Can you work these out from the model? Positions are in its coordinate system, mm. A direction names the side the tool comes from. Give positions to 0.01 mm unless a question says otherwise; leave off trailing zeros. Loops run counter-clockwise (first coordinate to the right, second up) from the corner with the lowest first, then second, coordinate; pieces in that order, holes last. Notation, with made-up numbers: (-20, -18.5) -> (37, -18.5) arc R7 ccw to (37, -5.5) -> close; hole circle Ø10 at (-35.5, 59.5). An arc over 180 degrees is marked (long way). Return JSON: item names as keys, results as strings. Group by question number.
Q1. I need wall thicknesses on line 1 along Z through (x, y) = (85, 1.75); line 2 along X through (y, z) = (2.95, -19); line 3 along X through (y, z) = (2.45, -25). Which ranges of each line are inside material? Lowest first, please. Write a range as [from, to].
Q2. Suppose I cut it at A-A, the plane x = 80.7. Please give me the cut outline in (y, z), and give its area (3 significant figures).
Q3. Which directions (+Z, -Z, +X, -X, +Y, -Y) give clear straight access to the entire face, cutting with the end or side of a thin tool? Please do faces 1 (the flat face through (59.7, 2, 0)), 2 (the flat face through (-1, 2, -60)).
Q4. Suppose I cut it at C-C, the plane y = 2.3. Count the separate pieces of the cut face and the enclosed holes in it, and give its area (3 significant figures).
Q5. Thinking about a two-plate mould opening in X: for faces 3 (the flat face through (-90, 2, 1)), 4 (the flat face through (39, 2, 15)), 5 (the flat face through (-1, 0, -1)), which applies, pulls with the +X half, pulls with the -X half, needs draft (parallel to the pull), parting line crosses it, or undercut?
Q6. Suppose I cut it at B-B, the plane z = -1. Please give me the cut outline in (x, y).
```python
from build123d import *

# Parameters (mm, degrees)
SKETCH_1_W          = 180
SKETCH_1_H          = 120
EXTRUDE_1_DEPTH     = 4
SKETCH_2_R          = 1.6
SKETCH_2_R_2        = 3
CUT_EXTRUDE_1_DEPTH = 4
SKETCH_3_W          = 40
SKETCH_3_H          = 30
CUT_EXTRUDE_2_DEPTH = 4
SKETCH_4_R          = 1.6
CUT_EXTRUDE_3_DEPTH = 4
SKETCH_5_R          = 1.6
CUT_EXTRUDE_4_DEPTH = 4


with BuildPart() as part:
    # 草图1 → 凸台-拉伸1 (new body)
    with BuildSketch(Plane(origin=(0, 0, 0), x_dir=(1, 0, 0), z_dir=(0, 1, 0))):
        Rectangle(SKETCH_1_W, SKETCH_1_H)
    extrude(amount=EXTRUDE_1_DEPTH)

    # 草图2 → 切除-拉伸1 (cut)
    with BuildSketch(Plane(origin=(0, 4, 0), x_dir=(1, 0, 0), z_dir=(0, 1, 0))):
        with Locations(Location((66, 25, 0), (0, 0, 270))):
            Circle(SKETCH_2_R)
        with Locations(Location((66, -25, 0), (0, 0, 270))):
            Circle(SKETCH_2_R)
        with Locations(Location((85, -25, 0), (0, 0, 270))):
            Circle(SKETCH_2_R)
        with Locations(Location((85, 25, 0), (0, 0, 270))):
            Circle(SKETCH_2_R)
        with Locations(Location((80.7, 7, 0), (0, 0, 270))):
            Circle(SKETCH_2_R_2)
    extrude(amount=-CUT_EXTRUDE_1_DEPTH, mode=Mode.SUBTRACT)

    # 草图3 → 切除-拉伸2 (cut)
    with BuildSketch(Plane(origin=(0, 4, 0), x_dir=(1, 0, 0), z_dir=(0, 1, 0))):
        with Locations((39.7, 0)):
            Rectangle(SKETCH_3_W, SKETCH_3_H)
    extrude(amount=-CUT_EXTRUDE_2_DEPTH, mode=Mode.SUBTRACT)

    # 草图4 → 切除-拉伸3 (cut)
    with BuildSketch(Plane(origin=(0, 4, 0), x_dir=(1, 0, 0), z_dir=(0, 1, 0))):
        with Locations(Location((-27.3, 56, 0), (0, 0, 270))):
            Circle(SKETCH_4_R)
        with Locations(Location((9.7, 56, 0), (0, 0, 270))):
            Circle(SKETCH_4_R)
        with Locations(Location((9.7, 19, 0), (0, 0, 270))):
            Circle(SKETCH_4_R)
        with Locations(Location((-27.3, 19, 0), (0, 0, 270))):
            Circle(SKETCH_4_R)
    extrude(amount=-CUT_EXTRUDE_3_DEPTH, mode=Mode.SUBTRACT)

    # 草图5 → 切除-拉伸4 (cut)
    with BuildSketch(Plane(origin=(0, 4, 0), x_dir=(1, 0, 0), z_dir=(0, 1, 0))):
        with Locations(Location((-39.8, -7.8, 0), (0, 0, 270))):
            Circle(SKETCH_5_R)
        with Locations(Location((9.7, -23, 0), (0, 0, 270))):
            Circle(SKETCH_5_R)
        with Locations(Location((9.7, -50.9, 0), (0, 0, 270))):
            Circle(SKETCH_5_R)
        with Locations(Location((-41.1, -56, 0), (0, 0, 270))):
            Circle(SKETCH_5_R)
    extrude(amount=-CUT_EXTRUDE_4_DEPTH, mode=Mode.SUBTRACT)


solid = part.part
```
Ans:
{
 "1": {"line 1": "z = [-60, -26.6], [-23.4, 23.4], [26.6, 60]", "line 2": "x = [-90, -28.9], [-25.7, 8.1], [11.3, 90]", "line 3": "x = [-90, 64.4], [67.6, 83.4], [86.6, 90]"},
 "2": {"outline": "(0, -60) -> (4, -60) -> (4, -10) -> (0, -10) -> close; (0, -4) -> (4, -4) -> (4, 60) -> (0, 60) -> close", "area": "456 mm^2"},
 "3": {"face 1": "+Y, -Y", "face 2": "-Z, +X, -X, +Y, -Y"},
 "4": {"separate pieces": "1", "enclosed holes": "14", "area": "20,300 mm^2"},
 "5": {"face 3": "pulls with the -X half", "face 4": "undercut", "face 5": "needs draft"},
 "6": {"outline": "(-90, 0) -> (19.7, 0) -> (19.7, 4) -> (-90, 4) -> close; (59.7, 0) -> (90, 0) -> (90, 4) -> (59.7, 4) -> close"}
}
